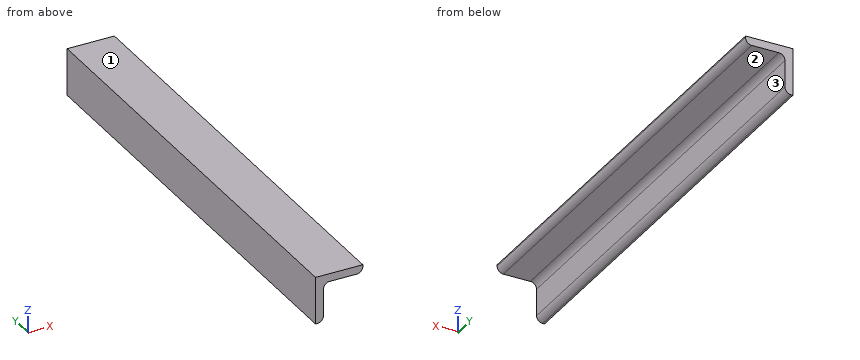
from build123d import *

# Parameters (mm, degrees)
F1_DEPTH = 370
F2_R     = 5
F3_R     = 5


with BuildPart() as f1:
    # F0 (on Front) → F1 (new body)
    with BuildSketch(Plane.XZ):
        Polygon((38, 0), (0, 0), (0, -38), (6.35, -38), (6.35, -6.343249), (38.292737, -6.343249), align=None)
    extrude(amount=F1_DEPTH)

    # F2
    f2_edges = [f1.edges().sort_by_distance(p)[0] for p in [
        (6.35, -185, -38),
        (6.35, -185, -6.343249),
    ]]
    fillet(f2_edges, radius=F2_R)

    # F3
    f3_edges = [f1.edges().sort_by_distance(p)[0] for p in [
        (38.292737, -185, -6.343249),
    ]]
    fillet(f3_edges, radius=F3_R)


solid = f1.part
The listing builds one solid part. Answer for the finished solid, in the listing's coordinates (mm). Face numbers are marked on the shaded views. Coordinates: 2 decimals unless noted, no trailing zeros. Loops run counter-clockwise (first coordinate to the right, second up) from the corner with the lowest first, then second, coordinate; pieces in that order, holes last.
1) Find the intervals of material crossed by L1, parallel to Z at x = 29.5, y = -283; L2, parallel to X at y = -338, z = -22.5, in increasing order.
2) Determine the mould class of the marked faces 1, 2 and 3 for opening direction Z: pulls with the +Z half, pulls with the -Z half, needs draft (parallel to the pull), parting line crosses it, or undercut.
3) Find section B-B on x = 27.5. Write down the section's boundary in (y, z).
4) Find section A-A on y = -302.5. Write down the section's boundary in (x, z).
5) Flat-ended cylindrical pins translate along their axes: pin 1 Ø12 at (y, z) = (-318, -16) entering from +X; pin 2 Ø1 at (y, z) = (-132, -13.5) entering from +X; pin 3 Ø4 at (y, z) = (-191.5, -32) entering from +X. Find the tip coordinate at first contact, or state that the pin passes through.
6) Find section C-C on z = -20. Write down the section's boundary in (x, y), then the cut area to 3 significant figures.
Values:
1. L1: z = -6.34 to 0
1. L2: x = 0 to 6.35
2. face 1: pulls with the +Z half
2. face 2: pulls with the -Z half
2. face 3: needs draft
3. outline: (-370, -6.34) - (0, -6.34) - (0, 0) - (-370, 0) - close
4. outline: (0, -38) - (1.35, -38) arc R5 ccw to (6.35, -33) - (6.35, -11.34) arc R5 cw to (11.35, -6.34) - (33.06, -6.34) arc R5 ccw to (38.05, -1.11) - (38, 0) - (0, 0) - close
5. pin 1: stops at x = 6.53
5. pin 2: stops at x = 6.35
5. pin 3: stops at x = 6.35
6. outline: (0, -370) - (6.35, -370) - (6.35, 0) - (0, 0) - close
6. area: 2,350 mm2
